Geometry check sheet. Reference: the model listing, model coordinates, mm. A direction names the side the tool comes from. Round coordinates to 2 decimals unless told otherwise and drop trailing zeros. Order: outer loops, then holes, each group sorted by start corner. A loop starts at its lowest first (then second) coordinate and runs counter-clockwise, first axis right, second up.
```python
from build123d import *

# Parameters (mm, degrees)
F0_W     = 1270
F0_H     = 1270
F1_DEPTH = 1000
F2_W     = 635
F2_H     = 626.05989
F3_DEPTH = 500
F5_DEPTH = 700


with BuildPart() as f1:
    # F0 (on Top) → F1 (new body)
    with BuildSketch(Plane.XY):
        with Locations((635, 635)):
            Rectangle(F0_W, F0_H)
    extrude(amount=F1_DEPTH)

    # F2 (on face) → F3 (cut)
    with BuildSketch(Plane.XY.offset(1000)):
        with Locations((317.5, 313.029945)):
            Rectangle(F2_W, F2_H)
    extrude(amount=-F3_DEPTH, mode=Mode.SUBTRACT)

    # F4 (on face) → F5 (cut)
    with BuildSketch(Plane(origin=(0, 1270, 0), x_dir=(-1, 0, 0), z_dir=(0, 1, 0))):
        Polygon((0, 1000), (-1270, 1000), (0, 0), align=None)
    extrude(amount=-F5_DEPTH, mode=Mode.SUBTRACT)


solid = f1.part
```
(1) Sectioned sample at B-B, the plane z = 897. Record the cut outline in (x, y).
Returned:
outline: (635, 0) - (1270, 0) - (1270, 1270) - (1139.19, 1270) - (1139.19, 570) - (635, 570) - close
(2) Material ranges on line 1 (X direction, y = 419.5, z = 949.5); line 2 (Z direction, x = 356, y = 557.5); line 3 (Y direction, x = 705, z = 706.5), recorded low to high.
Returned:
line 1: x = 635 to 1270
line 2: z = 0 to 500
line 3: y = 0 to 570
(3) Sectioned sample at C-C, the plane y = 965.5. Record the cut outline in (x, z).
Returned:
outline: (0, 0) - (1270, 0) - (1270, 1000) - close
(4) Set-up check for faces 1 (the flat face through (635, 281, 754)), 2 (the flat face through (1270, 626, 493)), 3 (the flat face through (181, 570, 365)): record each of +Z, -Z, +X, -X, +Y, -Y from which the full face is reachable in a straight line by a thin tool's end or side.
Returned:
face 1: +Z, -X, +Y, -Y
face 2: +Z, -Z, +X, +Y, -Y
face 3: +Z, -X, +Y
(5) Sectioned sample at A-A, the plane y = 363. Record the cut outline in (x, z), and give its area (4 significant figures).
Returned:
outline: (0, 0) - (1270, 0) - (1270, 1000) - (635, 1000) - (635, 500) - (0, 500) - close
area: 952,500 mm2
(6) Depth check by flat-ended pin: P1, Ø10, axis at x = 235, y = 542, coming from the +Z side; P2, Ø6, axis at y = 1052, z = 671, coming from the -X side; P3, Ø1.5, axis at x = 433.5, y = 781, coming from the +Z side. Enter the tip coordinate at first touch or a pass-through.
Returned:
P1: stops at z = 500
P2: stops at x = 848.36
P3: stops at z = 341.93
